```python
from build123d import *

# Parameters (mm, degrees)
BOSS_EXTRU_1_DEPTH      = 22.225
ESQUISSE2_R             = 9.525
ENL_V_MAT_EXTRU_1_DEPTH = 32.148999282


with BuildPart() as part:
    # Esquisse1 → Boss.-Extru.1 (new body)
    with BuildSketch(Plane(origin=(0, 0, 0), x_dir=(1, 0, 0), z_dir=(0, 1, 0))):
        Polygon((8.248891971, 14.2875), (-8.248891971, 14.2875), (-16.497783942, 0), (-8.248891971, -14.2875), (8.248891971, -14.2875), (16.497783942, 0), align=None)
    extrude(amount=BOSS_EXTRU_1_DEPTH)

    # Esquisse2 → Enlèv. mat.-Extru.1 (cut, through all)
    with BuildSketch(Plane(origin=(0, 22.225, 0), x_dir=(1, 0, 0), z_dir=(0, 1, 0))):
        with Locations(Location((0, 0, 0), (0, 0, 270))):
            Circle(ESQUISSE2_R)
    extrude(amount=-ENL_V_MAT_EXTRU_1_DEPTH, mode=Mode.SUBTRACT)

    # Esquisse3 → Enlèvement de matière-Révolution1 (revolve, cut)
    with BuildSketch(Plane(origin=(0, 0, 0), x_dir=(0, 0, -1), z_dir=(1, 0, 0)), mode=Mode.PRIVATE) as enl_vement_de_mati_re_r_volution1_sk:
        with BuildLine():
            Line((-14.2875, 22.225), (-12.7, 22.225))
            Line((-12.7, 22.225), (-11.1125, 22.225))
            ThreePointArc((-11.1125, 22.225), (-13.35756403, 21.29506403), (-14.2875, 19.05))
            Line((-14.2875, 19.05), (-17.4625, 19.05))
            Line((-17.4625, 19.05), (-17.4625, 22.225))
            Line((-17.4625, 22.225), (-14.2875, 22.225))
        make_face()
    revolve(enl_vement_de_mati_re_r_volution1_sk.sketch.rotate(Axis((0, 0, 0), (0, 1, 0)), 180), axis=Axis((0, 0, 0), (0, 1, 0)), mode=Mode.SUBTRACT)


solid = part.part
```
Input: part model. Units: mm. Frame: model coordinates. A direction names the side the tool comes from. Give positions to 0.01 mm unless a question says otherwise; leave off trailing zeros. Use a Markdown table: item, result.
(1) Access query for faces 1 (the flat face through (8, 19.05, 13)), 2 (the flat face through (8, 19.05, -13)), 3 (the flat face through (-7, 19.05, 13)), 4 (the flat face through (15, 19.05, 0)). Directions: +Z, -Z, +X, -X, +Y, -Y. A direction counts if a zero-diameter tool reaches every point of the face in a straight line with its end or side. Return the directions, or none.
Computed values:
| item | result |
|---|---|
| face 1 | +Z, +X, +Y |
| face 2 | -Z, +X, +Y |
| face 3 | +Z, -X, +Y |
| face 4 | +X, +Y |
(2) Pin query (flat end, axial travel): pin 1 (3.5 mm diameter, centred on x = -6, z = -12, fed in from +Y); pin 2 (2 mm diameter, centred on x = 15.5, z = -0.5, fed in from +Y); pin 3 (2 mm diameter, centred on x = 5, z = -12.5, fed in from +Y). Return the tip coordinate at first contact, or that it passes through.
Computed values:
| item | result |
|---|---|
| pin 1 | stops at y = 22.18 |
| pin 2 | stops at y = 19.05 |
| pin 3 | stops at y = 21.92 |
(3) Draft query along Z for faces 5 (the cylindrical face through (-5.796, 11.268, -7.559)), 6 (the flat face through (-7, 19.05, -13)), 7 (the flat face through (0, 9, 14.288)). Return one class per face: released by +Z, released by -Z, zero draft, split by the parting line, or undercut.
Computed values:
| item | result |
|---|---|
| face 5 | undercut |
| face 6 | zero draft |
| face 7 | released by +Z |
(4) Line query: line 1 (X direction, y = 9.25, z = 0) (3 decimals); line 2 (X direction, y = 16, z = -5.25); line 3 (Y direction, x = -2.5, z = 11). Output: solid intervals per line, ascending. Write a range as from..to.
Computed values:
| item | result |
|---|---|
| line 1 | x = -16.498..-9.525, 9.525..16.498 |
| line 2 | x = -13.47..-7.95, 7.95..13.47 |
| line 3 | y = 0..22.22 |
